Can you work these out from the model? Positions are in its coordinate system, mm. Face numbers are marked on the shaded views. A direction names the side the tool comes from. Coordinates: 2 decimals unless noted, no trailing zeros. Order: outer loops, then holes, each group sorted by start corner. A loop starts at its lowest first (then second) coordinate and runs counter-clockwise, first axis right, second up.
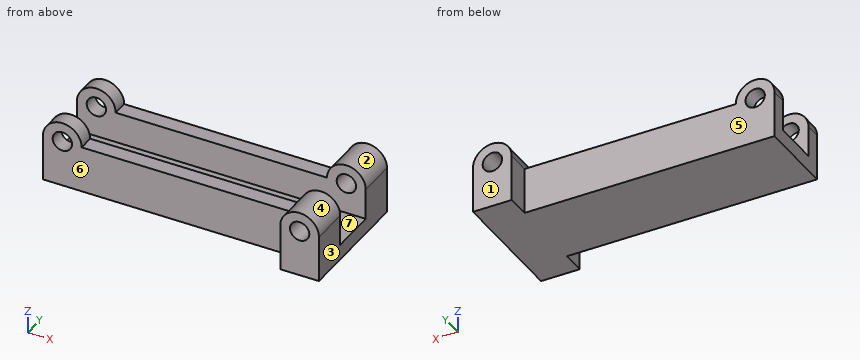
```python
from build123d import *

# Parameters (mm, degrees)
BOSS_EXTRUDE4_DEPTH = 6.35
SKETCH9_R           = 3.96875
BOSS_EXTRUDE5_DEPTH = 15.875
SKETCH10_R          = 3.96875
BOSS_EXTRUDE6_DEPTH = 6.35


with BuildPart() as part:
    # Sketch6 → Boss-Extrude4 (new body)
    with BuildSketch(Plane.XY):
        Polygon((0, 0), (0, -15.875), (102.5525, -15.875), (102.5525, -25.4), (118.4275, -25.4), (118.4275, 0), align=None)
    extrude(amount=BOSS_EXTRUDE4_DEPTH)

    # Sketch9 → Boss-Extrude5 (add)
    with BuildSketch(Plane.XZ.offset(25.4)):
        with BuildLine():
            Line((102.5525, 6.35), (102.5525, 19.05))
            ThreePointArc((102.5525, 19.05), (110.49, 26.9875), (118.4275, 19.05))
            Line((118.4275, 19.05), (118.4275, 6.35))
            Line((118.4275, 6.35), (102.5525, 6.35))
        make_face()
        with Locations(Location((110.49, 19.05, 0), (0, 0, 270))):
            Circle(SKETCH9_R, mode=Mode.SUBTRACT)
    extrude(amount=-BOSS_EXTRUDE5_DEPTH)

    # Sketch10 → Boss-Extrude6 (add)
    with BuildSketch(Plane.XZ.offset(15.875)):
        with BuildLine():
            Line((0, 6.35), (0, 19.05))
            ThreePointArc((0, 19.05), (7.9375, 26.9875), (15.875, 19.05))
            Line((15.875, 19.05), (102.5525, 19.05))
            Line((102.5525, 19.05), (102.5525, 6.35))
            Line((102.5525, 6.35), (0, 6.35))
        make_face()
        with Locations(Location((7.9375, 19.05, 0), (0, 0, 270))):
            Circle(SKETCH10_R, mode=Mode.SUBTRACT)
    extrude(amount=-BOSS_EXTRUDE6_DEPTH)

    # Mirror1: part across plane


with BuildPart() as part_1:
    add(part.part)
    add(part.part.mirror(Plane(origin=(118.4275, 0, 6.35), x_dir=(0, 0, 1), z_dir=(0, -1, 0))))


solid = part_1.part
```
1. I'm going to push flat-ended pins straight in: pin 1 (5 mm diameter, centred on x = 65, y = -18, fed in from +Z); pin 2 (5 mm diameter, centred on y = -22.5, z = 6, fed in from -X); pin 3 (1.5 mm diameter, centred on x = 25.5, z = 11, fed in from -Y) (3 decimals). Where does each tip first touch, or does it pass through?
Completed:
pin 1: stops at z = 19.05
pin 2: stops at x = 102.55
pin 3: stops at y = -15.875
2. Imagine slicing it at D-D on x = 80. Please give me the cut outline in (y, z) (3 decimals), then the cut area to 3 significant figures.
Completed:
outline: (-15.875, 0) - (15.875, 0) - (15.875, 19.05) - (9.525, 19.05) - (9.525, 6.35) - (-9.525, 6.35) - (-9.525, 19.05) - (-15.875, 19.05) - close
area: 363 mm2
3. Imagine slicing it at A-A on x = 110.49. Give the number of separate pieces and of enclosed holes in the cut face, then the cut area to 3 significant figures.
Completed:
separate pieces: 3
enclosed holes: 0
area: 726 mm2
4. On a 3-axis mill with a long thin cutter (end or side, diameter ignored), from which of +Z, -Z, +X, -X, +Y, -Y can I reach the whole of each face in a straight line? I mean the marked faces 5, 6 and 7. Say none if no direction works.
Completed:
face 5: +Z, -Z, -X, +Y
face 6: +Z, -Z, -X, -Y
face 7: +Z, +X, -X
5. Thinking about a two-plate mould opening in X: for the marked faces 1, 2, 3 and 4, which applies, pulls with the +X half, pulls with the -X half, needs draft (parallel to the pull), parting line crosses it, or undercut?
Completed:
face 1: needs draft
face 2: undercut
face 3: pulls with the +X half
face 4: undercut
6. Imagine slicing it at B-B on z = 9.5. Please give me the cut outline in (x, y) (1 decimal), then the cut area to 3 significant figures.
Completed:
outline: (0, -15.9) - (102.6, -15.9) - (102.6, -25.4) - (118.4, -25.4) - (118.4, -9.5) - (0, -9.5) - close; (0, 9.5) - (118.4, 9.5) - (118.4, 25.4) - (102.6, 25.4) - (102.6, 15.9) - (0, 15.9) - close
area: 1,810 mm2
7. Please list where these lines run through material, in increasing order: probe 1 along Y at (x, z) = (5, 8.25) (3 decimals); probe 2 along X at (y, z) = (15, 20); probe 3 along Y at (x, z) = (41.5, 3.5) (3 decimals).
Completed:
probe 1: y = -15.875 to -9.525, 9.525 to 15.875
probe 2: x = 0.06 to 4.08, 11.79 to 15.82, 102.61 to 106.64, 114.34 to 118.37
probe 3: y = -15.875 to 15.875
